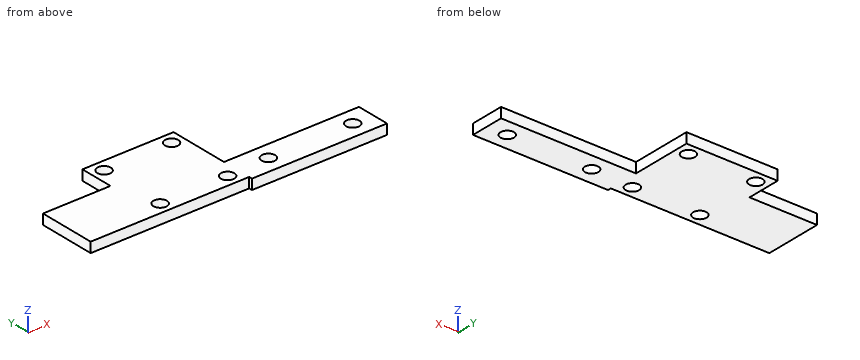
from build123d import *

# Parameters (mm, degrees)
F0_W     = 20
F0_H     = 20
F1_DEPTH = 3
F2_D     = 4
F0_H_2   = 7
F0_H_3   = 10
F3_DEPTH = 3


with BuildPart() as f1:
    # F0 (on Top) → F1 (new body)
    with BuildSketch(Plane.XY):
        Polygon((-13.5, -4), (13.5, -4), (13.5, 5), (13.5, 23), (-13.5, 23), (-13.5, 13), (-13.5, 6), align=None)
        with Locations((0, 9.5)):
            Rectangle(F0_W, F0_H, mode=Mode.SUBTRACT)
        with Locations((0, 9.5)):
            Rectangle(F0_W, F0_H)
        Polygon((13.5, 5), (13.5, -4), (13.5, -5), (53.5, -5), (53.5, 5), align=None)
    extrude(amount=-F1_DEPTH)

    # F2 (through all)
    with Locations(Plane.XY):
        with Locations((-10, -0.5), (-10, 19.5), (10, -0.5), (22.5, 0), (47.5, 0), (10, 19.5)):
            Hole(F2_D / 2)

    # F0 (on Top) → F3 (join)
    with BuildSketch(Plane.XY):
        with Locations((-23.5, 9.5)):
            Rectangle(F0_W, F0_H_2)
        with Locations((-23.5, 1)):
            Rectangle(F0_W, F0_H_3)
    extrude(amount=-F3_DEPTH)


solid = f1.part
Input: part model. Units: mm. Frame: model coordinates. Coordinates: 2 decimals unless noted, no trailing zeros. Order: outer loops, then holes, each group sorted by start corner. A loop starts at its lowest first (then second) coordinate and runs counter-clockwise, first axis right, second up. Notation, with made-up numbers: M 37.5,9.5 L 44.5,9.5 A20 ccw 44.5,24.5 Z; hole C 47,-19 d7. An arc over 180 degrees is marked long. Write item = value, one per line. Start each with the question number.
(1) Section C-C on x = 10. Output: boundary loops of the cut face in (y, z).
(2) First-contact query: P1, Ø5, axis at x = -16.5, y = 10, coming from the +Z side; P2, Ø1.5, axis at y = 13, z = -1, coming from the +X side; P3, Ø0.5, axis at y = -4.5, z = -1.5, coming from the -X side. Flat tips, straight axial feed; report the tip coordinate or a pass-through.
(3) Section B-B on z = -2.45. Output: boundary loops of the cut face in (x, y).
(4) Section D-D on x = 47.5. Output: boundary loops of the cut face in (y, z), and give its area (3 significant figures).
(5) Line query: line 1 along Y through (x, z) = (10, -0.6); line 2 along Y through (x, z) = (22.5, -0.8); line 3 along X through (y, z) = (21, -0.4). Output: solid intervals per line, ascending. Write a range as [from, to].
(6) Section A-A on y = 19.5. Output: boundary loops of the cut face in (x, z), and give its area (3 significant figures).
Result set:
q1.outline = M -4,-3 L -2.5,-3 L -2.5,0 L -4,0 Z; M 1.5,-3 L 17.5,-3 L 17.5,0 L 1.5,0 Z; M 21.5,-3 L 23,-3 L 23,0 L 21.5,0 Z
q2.P1 = 0
q2.P2 = 13.5
q2.P3 = 13.5
q3.outline = M -33.5,-4 L 13.5,-4 L 13.5,-5 L 53.5,-5 L 53.5,5 L 13.5,5 L 13.5,23 L -13.5,23 L -13.5,13 L -33.5,13 Z; hole C -10,-0.5 d4; hole C -10,19.5 d4; hole C 10,-0.5 d4; hole C 10,19.5 d4; hole C 22.5,0 d4; hole C 47.5,0 d4
q4.outline = M -5,-3 L -2,-3 L -2,0 L -5,0 Z; M 2,-3 L 5,-3 L 5,0 L 2,0 Z
q4.area = 18.0 mm²
q5.line_1 = [-4, -2.5], [1.5, 17.5], [21.5, 23]
q5.line_2 = [-5, -2], [2, 5]
q5.line_3 = [-13.5, -11.32], [-8.68, 8.68], [11.32, 13.5]
q6.outline = M -13.5,-3 L -12,-3 L -12,0 L -13.5,0 Z; M -8,-3 L 8,-3 L 8,0 L -8,0 Z; M 12,-3 L 13.5,-3 L 13.5,0 L 12,0 Z
q6.area = 57.0 mm²
